The listing builds one solid part. Answer for the finished solid, in the listing's coordinates (mm). Face numbers are marked on the shaded views. A direction names the side the tool comes from. Coordinates: 2 decimals unless noted, no trailing zeros. Order: outer loops, then holes, each group sorted by start corner. A loop starts at its lowest first (then second) coordinate and runs counter-clockwise, first axis right, second up. Notation, with made-up numbers: (76, 10) -> (109, 10) arc R6 cw to (109, 19) -> close; hole circle Ø1 at (34, 29). An arc over 180 degrees is marked (long way). Write item = value, one per line.
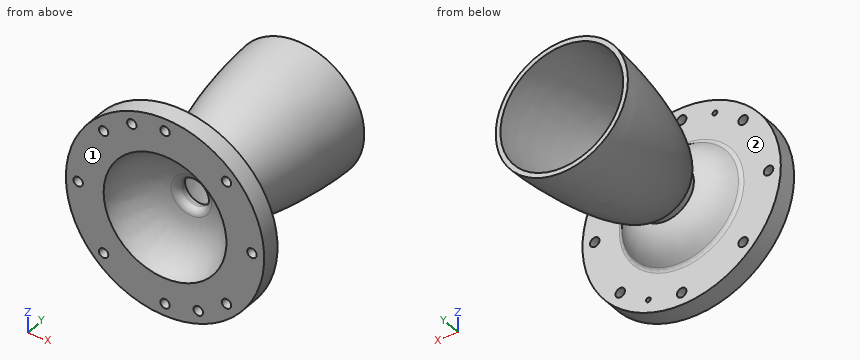
from build123d import *

# Parameters (mm, degrees)
CONVERGING_FILLET_R   = 3.175
BOLT_HOLES_D          = 6.35
BOLT_HOLES_DEPTH      = 12.7
BOLT_HOLES_TIP        = 1.907732465
PIN_HOLES_D           = 3.175
PIN_HOLES_DEPTH       = 100
PIN_HOLES_CBORE_D     = 6.35
PIN_HOLES_CBORE_DEPTH = 6.35


with BuildPart() as part:
    # Sketch1 → Main Revolve (revolve)
    with BuildSketch(Plane.XY):
        with BuildLine():
            Line((-9.517884855, 29.85426414), (-9.517884855, 31.004317662))
            ThreePointArc((-9.517884855, 31.004317662), (-10.387063469, 33.747209355), (-12.677340956, 35.488919819))
            add(Edge.make_bspline(
                [(-41.275, 127), (-41.268873036, 126.161357833), (-41.222997706, 124.484568363), (-41.073369126, 121.078528782), (-40.722786085, 115.949040077), (-40.170467422, 109.939618965), (-39.360849464, 103.059106185), (-38.382227863, 96.200616774), (-37.230570221, 89.368983139), (-35.895631241, 82.570619969), (-34.35912374, 75.814773558), (-32.593807355, 69.114550244), (-30.558516971, 62.490757957), (-28.191269221, 55.976383127), (-25.683140783, 50.29180013), (-23.125834222, 45.592543641), (-20.711209845, 42.055498174), (-18.720317843, 39.685916503), (-17.052831983, 38.103539579), (-15.746862259, 37.100217478), (-14.77072941, 36.476537732), (-14.077416444, 36.090491664), (-13.464775463, 35.797858298), (-13.037564762, 35.6215562), (-12.773284859, 35.523215456), (-12.677340956, 35.488919819)],
                knots=[0, 0, 0, 0, 0, 0.030811657, 0.061623313, 0.125250249, 0.188877076, 0.252503727, 0.31613061, 0.379757458, 0.443384315, 0.507011165, 0.570638032, 0.634264894, 0.697891611, 0.761518516, 0.798698062, 0.830511144, 0.855003573, 0.875012249, 0.882965592, 0.890918935, 0.897534321, 0.904149707, 0.907892787, 0.907892787, 0.907892787, 0.907892787, 0.907892787], degree=4))
            Line((-41.275, 127), (-44.449999999, 127))
            add(Edge.make_bspline(
                [(-44.449999999, 127), (-44.444048095, 126.089867786), (-44.399723494, 124.270031311), (-44.256170835, 120.604636062), (-43.921206973, 115.098603125), (-43.395046361, 108.666141993), (-42.624644612, 101.314791698), (-41.691159468, 93.9823601), (-40.588904101, 86.673339257), (-39.305520483, 79.393738689), (-37.819617038, 72.152599105), (-36.098890328, 64.963007024), (-34.092981802, 57.847082032), (-31.766198141, 50.972017381), (-29.315037347, 45.128649076), (-26.838138987, 40.469327818), (-24.570330265, 37.178251455), (-22.783120415, 35.132973657), (-21.307300799, 33.836487802), (-20.194653885, 33.074782772), (-19.515295281, 32.700466394), (-19.20577242, 32.548791321), (-19.05, 32.47725184)],
                knots=[0, 0, 0, 0, 0, 0.033160808, 0.066321616, 0.133644696, 0.20096779, 0.268290787, 0.335613842, 0.40293693, 0.470260007, 0.537583094, 0.604906139, 0.672229114, 0.739552316, 0.801869766, 0.835531618, 0.86410438, 0.88489762, 0.900577549, 0.906888404, 0.913134212, 0.913134212, 0.913134212, 0.913134212, 0.913134212], degree=4))
            Line((-19.05, 32.47725184), (-19.049955181, 28.041753321))
            add(Edge.make_bspline(
                [(-40.132928845, 12.7), (-40.083978858, 12.784156262), (-39.983265103, 12.955401456), (-39.759808639, 13.330999271), (-39.546364559, 13.67507087), (-39.221651837, 14.190368882), (-38.914624104, 14.656083798), (-38.583549151, 15.143878505), (-38.186353269, 15.705830102), (-37.77509929, 16.268618988), (-37.2843995, 16.909714234), (-36.702796259, 17.630765959), (-36.103434504, 18.334481647), (-35.484819509, 19.022919017), (-34.848061727, 19.693649754), (-34.192734181, 20.346852672), (-33.519373114, 20.981085312), (-32.827952052, 21.595818623), (-31.962967273, 22.320542927), (-31.070351962, 23.011417112), (-30.150953105, 23.666133634), (-29.205505922, 24.282436301), (-28.414577383, 24.76223971), (-27.607968747, 25.215620128), (-26.786861464, 25.641439606), (-25.950949864, 26.038789389), (-25.102603979, 26.406415537), (-24.239975487, 26.743680196), (-23.368438554, 27.049008091), (-22.48141889, 27.322515066), (-21.704602088, 27.531618066), (-21.021032253, 27.69122915), (-20.468248248, 27.807088311), (-19.986741847, 27.896157232), (-19.629776323, 27.957756939), (-19.260320361, 28.012378489), (-19.106911701, 28.033992962), (-19.049955181, 28.041753321)],
                knots=[0.073786485, 0.073786485, 0.073786485, 0.073786485, 0.073786485, 0.088217084, 0.102647684, 0.117078284, 0.131508883, 0.160370079, 0.174800677, 0.189231275, 0.218092486, 0.246953697, 0.275814909, 0.304676121, 0.333537325, 0.362398529, 0.391259738, 0.420120946, 0.448982156, 0.477843365, 0.532083348, 0.560944559, 0.589805767, 0.618666976, 0.647528184, 0.676389393, 0.705250602, 0.734111807, 0.762973012, 0.79183422, 0.820695429, 0.849556636, 0.863987238, 0.87841784, 0.892848442, 0.907279044, 0.915799347, 0.915799347, 0.915799347, 0.915799347, 0.915799347], degree=4))
            Line((-40.132928845, 12.7), (-66.675, 12.7))
            Line((-66.675, 12.7), (-66.675, 0))
            Line((-66.675, 0), (-41.275, 0))
            add(Edge.make_bspline(
                [(-41.275, 0), (-41.27404827, 0.048633732), (-41.270265816, 0.145822286), (-41.249886429, 0.420698051), (-41.184454538, 0.952068232), (-41.045697232, 1.718226005), (-40.803050388, 2.710615824), (-40.471359514, 3.795919992), (-40.073863441, 4.892829094), (-39.58250679, 6.074812663), (-38.909330489, 7.49520986), (-38.013176032, 9.129802593), (-36.850990459, 10.946036297), (-35.454742127, 12.816921248), (-33.931439219, 14.585782904), (-32.290383905, 16.245919147), (-30.54007116, 17.790421623), (-28.688732636, 19.212251207), (-26.744575764, 20.504343604), (-24.716209135, 21.659734331), (-22.61250234, 22.671709773), (-20.443220111, 23.533972634), (-18.496293348, 24.152467466), (-16.799886455, 24.58239915), (-15.513443264, 24.843608525), (-14.65819574, 24.990901269), (-14.086451577, 25.07519752), (-13.804404299, 25.113562074), (-13.666257288, 25.131526207)],
                knots=[0, 0, 0, 0, 0, 0.004014849, 0.008029698, 0.022747096, 0.044177712, 0.068247366, 0.092316927, 0.116386463, 0.140456137, 0.173883837, 0.222022894, 0.270162138, 0.318301135, 0.366440287, 0.41457937, 0.462718533, 0.510857613, 0.558996755, 0.607135854, 0.655274938, 0.703414059, 0.751553162, 0.775622711, 0.799692261, 0.811727037, 0.823244082, 0.823244082, 0.823244082, 0.823244082, 0.823244082], degree=4))
            ThreePointArc((-13.666257288, 25.131526207), (-10.702243662, 26.711285957), (-9.517884855, 29.85426414))
        make_face()
    revolve(axis=Axis((0, 0, 0), (0, 1, 0)))

    # Converging Fillet
    converging_fillet_edges = [part.edges().sort_by_distance(p)[0] for p in [
        (40.132928845, 12.7, 0),
    ]]
    fillet(converging_fillet_edges, radius=CONVERGING_FILLET_R)

    # Bolt Holes
    with Locations(Plane(origin=(0, 12.7, 0), x_dir=(1, 0, 0), z_dir=(0, 1, 0))):
        with Locations((-58.42, 0), (-41.309178157, 41.309178157), (0, 58.42), (41.309178157, 41.309178157), (58.42, 0), (41.309178157, -41.309178157), (0, -58.42), (-41.309178157, -41.309178157)):
            Hole(BOLT_HOLES_D / 2, depth=BOLT_HOLES_DEPTH)
            with Locations((0, 0, -(BOLT_HOLES_DEPTH + BOLT_HOLES_TIP / 2))):  # 118° drill point
                Cone(0, BOLT_HOLES_D / 2, BOLT_HOLES_TIP, mode=Mode.SUBTRACT)

    # Pin Holes
    with Locations(Plane(origin=(0, 0, 0), x_dir=(-1, 0, 0), z_dir=(0, -1, 0))):
        with Locations((-22.356366119, 53.973042289), (22.356366119, -53.973042289)):
            CounterBoreHole(PIN_HOLES_D / 2, PIN_HOLES_CBORE_D / 2, PIN_HOLES_CBORE_DEPTH, depth=PIN_HOLES_DEPTH)


solid = part.part
Q1. Section A-A, the plane x = 58.42 is taken. Give the vertices of the cut face in (y, z) (3 decimals).
The answers:
outline = (0, -32.135) -> (12.7, -32.135) -> (12.7, -3.175) -> (0, -3.175) -> close; (0, 3.175) -> (12.7, 3.175) -> (12.7, 32.135) -> (0, 32.135) -> close
Q2. Find the intervals of material crossed by line 1 along Z through (x, y) = (0, 30.45); line 2 along X through (y, z) = (109, 25); line 3 along Y through (x, z) = (-20, 12), in increasing order.
The answers:
line_1 = -19.05 to -9.52, 9.52 to 19.05
line_2 = -35.46 to -31.27, 31.27 to 35.46
line_3 = 22.31 to 27.06, 35.8 to 46.12
Q3. Section B-B, the plane x = 0 is taken. Give the number of separate pieces and of enclosed holes in the cut face, plus the area to 3 significant figures.
The answers:
separate_pieces = 4
enclosed_holes = 0
area = 1,770 mm2
Q4. A tool of negligible diameter and unlimited length cuts with its end or side. For the marked faces 1 and 2, from which of +Z, -Z, +X, -X, +Y, -Y can it reach the whole face along a straight path? Write none if from no direction.
The answers:
face_1 = +Z, -Z, +X, -X, -Y
face_2 = none
Q5. Each of these flat-tipped pins is pushed along its axis until it touches: pin 1 Ø8.5 at (x, z) = (22.36, -53.97) entering from +Y; pin 2 Ø8 at (x, y) = (34.5, 108.5) entering from -Z; pin 3 Ø4 at (x, z) = (-22.36, 53.97) entering from -Y; pin 4 Ø4 at (x, z) = (-41.31, -41.31) entering from -Y. Where does it stop, or does it pass through?
The answers:
pin_1 = 12.7
pin_2 = -30.83
pin_3 = 6.35
pin_4 = through
